Autodesk Inventor part; units mm, degrees
ref_plane "YZ Plane" through (0, 0, 0) normal (1, 0, 0) x (0, 1, 0)
ref_plane "XZ Plane" through (0, 0, 0) normal (0, 1, 0) x (-1, 0, 0)
ref_plane "XY Plane" through (0, 0, 0) normal (0, 0, 1) x (1, 0, 0)
sketch "Sketch1" plane through (0, 0, 0) normal (0, 1, 0) x (-1, 0, 0)
  line L0 (0, 0) -> (-16.51, 0)
  line L1 (-16.51, 0) -> (-16.51, -7.62)
  line L2 (-16.51, -7.62) -> (0, -7.62)
  line L3 (0, -7.62) -> (0, 0)
  line L4 (-8.255, 0) -> (-5.715, 0)
  line L5 (-5.715, 0) -> (-5.715, 6.35)
  line L6 (-5.715, 6.35) -> (-10.795, 6.35)
  line L7 (-10.795, 6.35) -> (-10.795, 0)
  line L8 (-5.715, -7.62) -> (-5.715, -8.89)
  line L9 (-5.715, -8.89) -> (-10.795, -8.89)
  line L10 (-10.795, -8.89) -> (-10.795, -7.62)
  line L11 (-10.795, 6.35) -> (-10.795, 3.81)
  line L12 (-10.795, 3.81) -> (-13.335, 3.81)
  line L13 (-13.335, 3.81) -> (-10.795, 6.35)
  line L14 (-5.715, 6.35) -> (-5.715, 3.81)
  line L15 (-5.715, 3.81) -> (-3.175, 3.81)
  line L16 (-3.175, 3.81) -> (-5.715, 6.35)
  point P0 (-8.255, -7.62)
  point P1 (0, -3.81)
  point P2 (-16.51, -3.81)
  dimension "d0" = 16.51
  dimension "d1" = 7.62
  dimension "d2" = 2.54
  dimension "d3" = 6.35
  dimension "d4" = 5.08
  dimension "d5" = 1.27
  dimension "d6" = 2.54
  dimension "d7" = 2.54
  dimension "d8" = 2.54
  dimension "d9" = 2.54
extrude "Extrusion1" add sketch "Sketch1" along normal blind 38.1
sketch "Sketch2" plane through (0, 38.1, 0) normal (0, 1, 0) x (1, 0, 0)
  line L0 (16.51, 0) -> (16.51, 7.62)
  line L1 (16.51, 3.81) -> (12.7, 3.81)
  line L2 (0, 7.62) -> (0, 0)
  circle A0 centre (12.7, 3.81) radius 1.016
  dimension "d12" = 3.81
  dimension "d14" = 2.032
extrude "Extrusion2" add sketch "Sketch2" along normal blind 1.27
sketch "Sketch3" plane through (0, 38.1, 0) normal (0, 1, 0) x (1, 0, 0)
  line L0 (0, 7.62) -> (0, 0)
  line L1 (0, 3.81) -> (3.81, 3.81)
  circle A0 centre (3.81, 3.81) radius 1.016
  dimension "d20" = 3.81
  dimension "d21" = 2.032
extrude "Extrusion3" add sketch "Sketch3" along normal blind 1.27
sketch "Sketch6" plane through (0, 38.1, 0) normal (0, 1, 0) x (1, 0, 0)
  line L0 (16.51, 0) -> (16.51, 7.62)
  line L1 (16.51, 3.81) -> (8.255, 3.81)
  circle A0 centre (8.255, 3.81) radius 1.397
  point P0 (0, 0)
  dimension "d24" = 8.255
  dimension "d25" = 2.794
hole "Hole1" at (8.255, 38.1, -3.81) at (8.255, 38.1, -3.81) direction (0, -1, 0) diameter 2.794 depth 11.43 tip angle 118
sketch "Sketch13" plane through (0, 0, -7.62) normal (-1, 0, 0) x (0, 0, 1)
  line L0 (0, 0) -> (0, 38.1)
  line L1 (0, 0) -> (5.588, 0)
  line L2 (5.588, 0) -> (5.588, 10.16)
  line L3 (5.588, 10.16) -> (0, 10.16)
  line L4 (0, 10.16) -> (0, 0)
  point P0 (7.62, 0)
  dimension "d68" = 5.588
  dimension "d69" = 10.16
extrude "Extrusion7" add sketch "Sketch13" along normal blind 12.7
sketch "Sketch14" plane through (0, 0, -2.032) normal (0, 0, 1) x (1, 0, 0)
  line L0 (-12.7, 10.16) -> (-12.7, 0)
  line L1 (-12.7, 0) -> (-6.35, 0)
  line L2 (-6.35, 0) -> (-6.35, 10.16)
  line L3 (-6.35, 10.16) -> (-12.7, 10.16)
  line L4 (-12.7, 10.16) -> (-12.7, 0)
  point P0 (0, 0)
  dimension "d72" = 6.35
  dimension "d73" = 10.16
extrude "Extrusion8" add sketch "Sketch14" along normal blind 22.606
sketch "Sketch15" plane through (0, 0, 20.574) normal (0, 0, 1) x (1, 0, 0)
  line L0 (-12.7, 10.16) -> (-12.7, 0)
  line L1 (-12.7, 5.08) -> (-9.525, 5.08)
  circle A0 centre (-9.525, 5.08) radius 2.032
  point P0 (0, 0)
  dimension "d79" = 3.175
  dimension "d80" = 4.064
extrude "Extrusion9" add sketch "Sketch15" along normal blind 5.08
sketch "Sketch16" plane through (-9.525, 5.08, 25.654) normal (0, 0, 1) x (1, 0, 0)
  point P0 (9.525, -5.08)
sketch "Sketch17" plane through (-9.525, 5.08, 25.654) normal (0, 0, 1) x (1, 0, 0)
  circle A0 centre (0, 0) radius 1.397
  point P0 (9.525, -5.08)
  dimension "d83" = 2.794
hole "Hole3" at (-9.525, 5.08, 25.654) direction (0, 0, -1) diameter 2.794 depth 12.7 tip angle 118
sketch "Sketch18" plane through (10.795, 0, -8.89) normal (0, 0, -1) x (-1, 0, 0)
  line L0 (0, 0) -> (5.08, 0)
  line L1 (0, 38.1) -> (5.08, 38.1)
  line L2 (5.08, 38.1) -> (5.08, 0)
  line L3 (5.08, 0) -> (0, 0)
  line L4 (0, 0) -> (0, 38.1)
  point P0 (10.795, 0)
extrude "Extrusion10" cut sketch "Sketch18" against normal blind 1.27
properties part number "Grab1"
Design review of the part built by this model. Coordinates are the model's own, in mm. A direction names the side the tool comes from. Give positions to 0.01 mm unless a question says otherwise; leave off trailing zeros. Order: outer loops, then holes, each group sorted by start corner. A loop starts at its lowest first (then second) coordinate and runs counter-clockwise, first axis right, second up. Notation, with made-up numbers: (-25.5, -30) - (13.5, -30) arc R15 ccw to (13.5, -19) - close; hole circle Ø11 at (-17, -33). An arc over 180 degrees is marked (long way). Use a Markdown table: item, result. Add a question column.
(1) Add section D-D on z = 20. Give the boundary of the cut face in (x, y) (3 decimals), then the cut area to 3 significant figures.
(2) Machinability: for faces 5 (the face through (-9, 10.16, 3)), 6 (the face through (13.669, 38.726, -3.505)), 7 (the face through (5.715, 19, 2)), which of the approach directions +Z, -Z, +X, -X, +Y, -Y give a long, thin tool a straight path to every point of the face, cutting with its end or side? Answer none if there is none.
(3) Add section C-C on y = 20. Give the boundary of the cut face in (x, z) (3 decimals).
(4) Clearance check with flat-ended pins moving along their axes: P1, Ø6, axis at y = 17, z = -5.5, coming from the -X side; P2, Ø7, axis at x = -9.5, y = 4.5, coming from the +Z side; P3, Ø4.5, axis at x = 13.5, y = 14.5, coming from the +Z side (3 decimals); P4, Ø1.9, axis at y = 25, z = 2, coming from the +X side (3 decimals). State where each tip first meets the part, or that it passes through.
(5) Mouldability with a two-part tool opening along Y and no side actions: class faces 1 (the face through (-7.587, 4.47, 23.078)), 2 (the face through (4.427, 18.783, 5.062)), 3 (the face through (-9.945, 3.748, 19.215)), 4 (the face through (4, 39.37, -4)) as +Y half, -Y half, draft (parallel to the pull), parting line (faces both ways), or undercut.
(6) Wall thickness on probe 1 along X at (y, z) = (32, -3.81); probe 2 along X at (y, z) = (5, 20); probe 3 along Y at (x, z) = (-10, 20): over which ranges is each line inside the solid? List them lowest first. Write a range as [from, to].
(7) Add section B-B on x = 3.81. Give the boundary of the cut face in (y, z) (3 decimals).
(8) Add section A-A on z = 0.5. Give the boundary of the cut face in (x, y) (3 decimals), then the cut area to 3 significant figures.
Report:
| question | item | result |
|---|---|---|
| 1 | outline | (-12.7, 0) - (-6.35, 0) - (-6.35, 10.16) - (-12.7, 10.16) - close; hole circle Ø2.794 at (-9.525, 5.08) |
| 1 | area | 58.4 mm² |
| 2 | face 5 | +Z, -Z, -X, +Y |
| 2 | face 6 | +Y |
| 2 | face 7 | +Y, -Y |
| 3 | outline | (0, -7.62) - (16.51, -7.62) - (16.51, 0) - (10.795, 0) - (10.795, 3.81) - (13.335, 3.81) - (10.795, 6.35) - (5.715, 6.35) - (3.175, 3.81) - (5.715, 3.81) - (5.715, 0) - (0, 0) - close |
| 4 | P1 | stops at x = 0 |
| 4 | P2 | stops at z = 25.65 |
| 4 | P3 | stops at z = 5.895 |
| 4 | P4 | stops at x = 10.795 |
| 5 | face 1 | parting line |
| 5 | face 2 | draft |
| 5 | face 3 | undercut |
| 5 | face 4 | +Y half |
| 6 | probe 1 | x = [0, 6.86], [9.65, 16.51] |
| 6 | probe 2 | x = [-12.7, -10.92], [-8.13, -6.35] |
| 6 | probe 3 | y = [0, 3.77], [6.39, 10.16] |
| 7 | outline | (0, -7.62) - (38.1, -7.62) - (38.1, -4.826) - (39.37, -4.826) - (39.37, -2.794) - (38.1, -2.794) - (38.1, 0) - (0, 0) - close; (0, 3.81) - (38.1, 3.81) - (38.1, 4.445) - (0, 4.445) - close |
| 8 | outline | (-12.7, 0) - (-6.35, 0) - (-6.35, 10.16) - (-12.7, 10.16) - close; (5.715, 0) - (10.795, 0) - (10.795, 38.1) - (5.715, 38.1) - close |
| 8 | area | 258 mm² |
